Part model, mm, in its own coordinate system. Give positions to 0.01 mm unless a question says otherwise; leave off trailing zeros. Order: outer loops, then holes, each group sorted by start corner. A loop starts at its lowest first (then second) coordinate and runs counter-clockwise, first axis right, second up. Notation, with made-up numbers: (20.25, 43) -> (30.25, 43) arc R17 cw to (30.25, 55) -> close; hole circle Ø10 at (59.25, 48.25). An arc over 180 degrees is marked (long way). Write item = value, one per line. Start each with the question number.
Item 1: Band-saw the part on B-B on y = -1. Write the cut outline in (x, z).
Item 2: Band-saw the part on A-A on z = 107.5. Write the cut outline in (x, y), plus the area to 3 significant figures.
Item 3: Drill centre lines: line 1 along Y through (x, z) = (1.25, 51); line 2 along X through (y, z) = (5.7, 200). Where is each one in solid material? Low to high.
```python
from build123d import *

# Parameters (mm, degrees)
SKETCH_1_W          = 12
SKETCH_1_H          = 12
SKETCH_1_W_2        = 10
SKETCH_1_H_2        = 10
EXTRUDE_1_DEPTH     = 400
SKETCH_2_R          = 2.1
CUT_EXTRUDE_1_DEPTH = 500
SKETCH_3_R          = 2.1
CUT_EXTRUDE_2_DEPTH = 102


with BuildPart() as part:
    # 草图1 → 凸台-拉伸1 (new body)
    with BuildSketch(Plane.XY):
        Rectangle(SKETCH_1_W, SKETCH_1_H)
        Rectangle(SKETCH_1_W_2, SKETCH_1_H_2, mode=Mode.SUBTRACT)
    extrude(amount=EXTRUDE_1_DEPTH)

    # 草图2 → 切除-拉伸1 (cut)
    with BuildSketch(Plane(origin=(0, 6, 0), x_dir=(1, 0, 0), z_dir=(0, 1, 0))):
        with Locations(Location((0, -200, 0), (0, 0, 180))):
            Circle(SKETCH_2_R)
        with Locations(Location((0, -227, 0), (0, 0, 180))):
            Circle(SKETCH_2_R)
        with Locations(Location((0, -254, 0), (0, 0, 180))):
            Circle(SKETCH_2_R)
        with Locations(Location((0, -281, 0), (0, 0, 180))):
            Circle(SKETCH_2_R)
        with Locations(Location((0, -308, 0), (0, 0, 180))):
            Circle(SKETCH_2_R)
        with Locations(Location((0, -335, 0), (0, 0, 180))):
            Circle(SKETCH_2_R)
        with Locations(Location((0, -173, 0), (0, 0, 180))):
            Circle(SKETCH_2_R)
        with Locations(Location((0, -146, 0), (0, 0, 180))):
            Circle(SKETCH_2_R)
        with Locations(Location((0, -119, 0), (0, 0, 180))):
            Circle(SKETCH_2_R)
        with Locations(Location((0, -92, 0), (0, 0, 180))):
            Circle(SKETCH_2_R)
        with Locations(Location((0, -65, 0), (0, 0, 180))):
            Circle(SKETCH_2_R)
    extrude(amount=-CUT_EXTRUDE_1_DEPTH, mode=Mode.SUBTRACT)

    # 草图3 → 切除-拉伸2 (cut)
    with BuildSketch(Plane(origin=(0, 6, 0), x_dir=(1, 0, 0), z_dir=(0, 1, 0))):
        with Locations(Location((0, -6.5, 0), (0, 0, 180))):
            Circle(SKETCH_3_R)
        with Locations(Location((0, -26.5, 0), (0, 0, 180))):
            Circle(SKETCH_3_R)
        with Locations(Location((0, -373.5, 0), (0, 0, 180))):
            Circle(SKETCH_3_R)
        with Locations(Location((0, -393.5, 0), (0, 0, 180))):
            Circle(SKETCH_3_R)
    extrude(amount=-CUT_EXTRUDE_2_DEPTH, mode=Mode.SUBTRACT)


solid = part.part
```
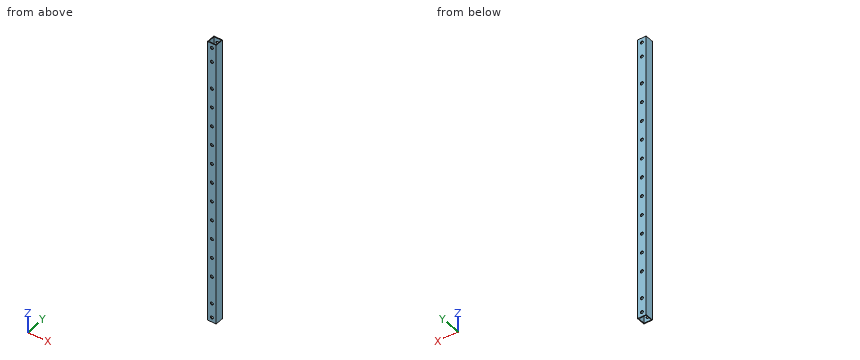
Values found:
q1.outline = (-6, 0) -> (-5, 0) -> (-5, 400) -> (-6, 400) -> close; (5, 0) -> (6, 0) -> (6, 400) -> (5, 400) -> close
q2.outline = (-6, -6) -> (6, -6) -> (6, 6) -> (-6, 6) -> close; hole (-5, -5) -> (5, -5) -> (5, 5) -> (-5, 5) -> close
q2.area = 44.0 mm^2
q3.line_1 = -6 to -5, 5 to 6
q3.line_2 = -6 to -2.1, 2.1 to 6
